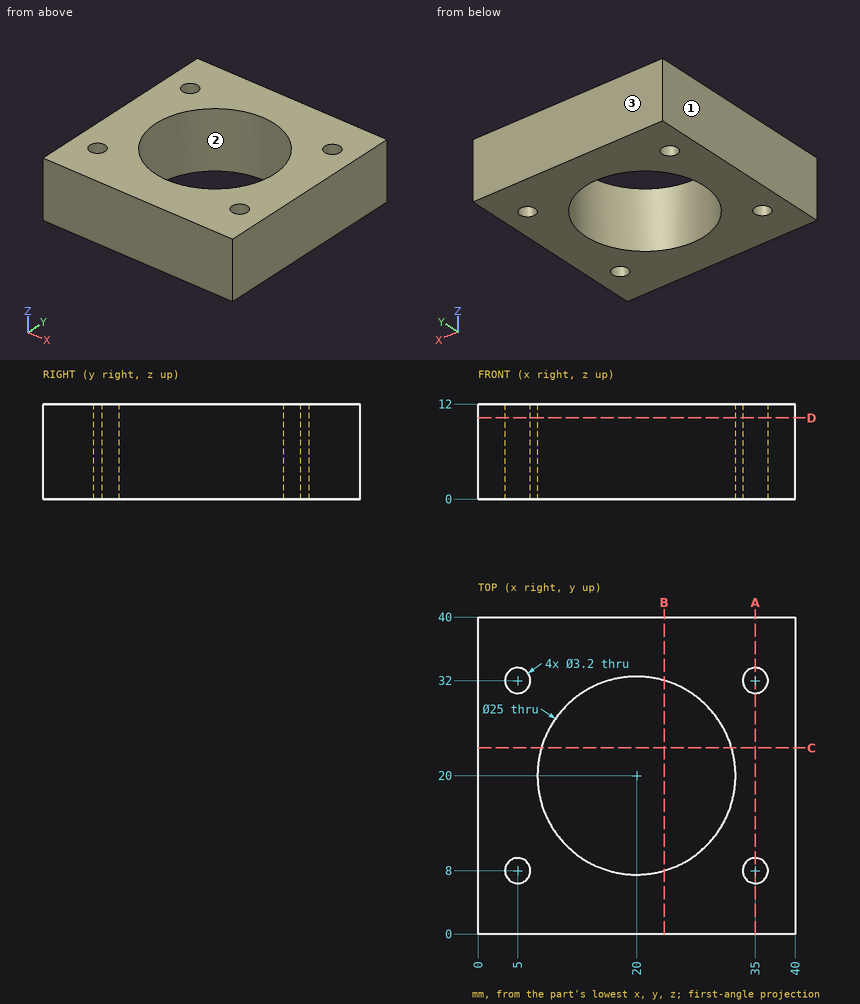
Study the drawing (mm; zero at the part's minimum x, y, z) and answer. Give positions to 0.01 mm unless a question says otherwise; leave off trailing zeros. Order: outer loops, then holes, each group sorted by start corner. A loop starts at its lowest first (then second) coordinate and runs counter-clockwise, first axis right, second up.
1. The mould has two halves that part along Y. Classify the marked faces 1, 2 and 3: released by +Y, released by -Y, zero draft, split by the parting line, or undercut.
Result sheet:
face 1: zero draft
face 2: undercut
face 3: released by +Y
2. Section B-B, the plane x = 23.5 is taken. Determine the outline of the cut face in (y, z), and give its area (3 significant figures).
Result sheet:
outline: (0, 0) - (8, 0) - (8, 12) - (0, 12) - close; (32, 0) - (40, 0) - (40, 12) - (32, 12) - close
area: 192 mm2
3. Section D-D, the plane z = 10.25 is taken. Determine the outline of the cut face in (x, y).
Result sheet:
outline: (0, 0) - (40, 0) - (40, 40) - (0, 40) - close; hole circle Ø3.2 at (5, 8); hole circle Ø3.2 at (5, 32); hole circle Ø25 at (20, 20); hole circle Ø3.2 at (35, 8); hole circle Ø3.2 at (35, 32)
4. Straight lines are drawn through the part: L1, parallel to Y at x = 35, z = 7; L2, parallel to Y at x = 4, z = 11.25; L3, parallel to X at y = 31, z = 5.5. For each, find the intervals that lie inside material, in ascending order.
Result sheet:
L1: y = 0 to 6.4, 9.6 to 30.4, 33.6 to 40
L2: y = 0 to 6.75, 9.25 to 30.75, 33.25 to 40
L3: x = 0 to 3.75, 6.25 to 14.06, 25.94 to 33.75, 36.25 to 40
5. Section A-A, the plane x = 35 is taken. Determine the outline of the cut face in (y, z), and give its area (3 significant figures).
Result sheet:
outline: (0, 0) - (6.4, 0) - (6.4, 12) - (0, 12) - close; (9.6, 0) - (30.4, 0) - (30.4, 12) - (9.6, 12) - close; (33.6, 0) - (40, 0) - (40, 12) - (33.6, 12) - close
area: 403 mm2
